For this review, take the finished solid that the model builds, in its own axes (mm). Face numbers are marked on the shaded views. A direction names the side the tool comes from. Coordinates: 2 decimals unless noted, no trailing zeros.
1. Machinability: for the marked faces 1 and 2, which of the approach directions +Z, -Z, +X, -X, +Y, -Y give a long, thin tool a straight path to every point of the face, cutting with its end or side? Answer none if there is none.
2. Clearance check with flat-ended pins moving along their axes: P1, Ø12, axis at y = -27, z = -39.5, coming from the +X side; P2, Ø1.5, axis at y = -68, z = 23, coming from the +X side; P3, Ø1.2, axis at y = 6.5, z = 12, coming from the +X side; P4, Ø12, axis at x = 10, z = -38.5, coming from the -Y side. State where each tip first meets the part, or that it passes through.
3. Mouldability with a two-part tool opening along Y and no side actions: class the marked faces 3 and 4 as pulls with the +Y half, pulls with the -Y half, needs draft (parallel to the pull), parting line crosses it, or undercut.
4. To check wall thickness, follow probe 1 along X at (y, z) = (51.5, -46.5); probe 2 along Y at (x, z) = (-2, -27); probe 3 along Z at (x, y) = (-1, 8.5). State the ranges of each line that lie inside material, in increasing order.
5. Take a section at A-A, the plane y = -26. Count the separate pieces of the cut face and the enclosed holes in it, then the cut area to 3 significant figures.
```python
from build123d import *

# Parameters (mm, degrees)
F0_R     = 85
F0_R_2   = 60.1341050947
F1_DEPTH = 10
F0_R_3   = 5
F0_R_4   = 18.4571799951
F2_DEPTH = 2.5
F3_DEPTH = 10
F4_R     = 5
F0_R_5   = 7.4694808043
F6_DEPTH = 20


# Not quite as in the source:
# - a fillet or chamfer that OpenCascade refuses, or shapes differently, is made with other operations: its cross-section is extruded or revolved along the edge and cut away or added


with BuildPart() as f1:
    # F0 (on Right) → F1 (new body, symmetric)
    with BuildSketch(Plane.YZ):
        Circle(F0_R)
        Circle(F0_R_2, mode=Mode.SUBTRACT)
    extrude(amount=F1_DEPTH, both=True)

    # F0 (on Right) → F2 (join, symmetric)
    with BuildSketch(Plane.YZ):
        Circle(F0_R_2)
        with Locations((-25.7258657366, -25.725863874)):
            Circle(F0_R_3, mode=Mode.SUBTRACT)
        with Locations((26.0370634496, -26.0024871677)):
            Circle(F0_R_3, mode=Mode.SUBTRACT)
        with Locations((-26, 26)):
            Circle(F0_R_3, mode=Mode.SUBTRACT)
        Circle(F0_R_4, mode=Mode.SUBTRACT)
        with Locations((26.2791067362, 26.2791085988)):
            Circle(F0_R_3, mode=Mode.SUBTRACT)
    extrude(amount=F2_DEPTH, both=True)

    # F0 (on Right) → F3 (join, symmetric)
    with BuildSketch(Plane.YZ):
        Circle(F0_R_4)
        Polygon((12.8988242803, 8.4499999602), (13.7673267676, -6.9457095256), (0.8685024874, -15.3957094858), (-12.8988242803, -8.4499999602), (-13.7673267676, 6.9457095256), (-0.8685024874, 15.3957094858), align=None, mode=Mode.SUBTRACT)
    extrude(amount=F3_DEPTH, both=True)

    # F4
    f4_edges = [f1.edges().sort_by_distance(p)[0] for p in [
        (-10, -85, 0),
        (10, -85, 0),
    ]]
    fillet(f4_edges, radius=F4_R)

    # F5: chamfer of 5 on 2 edges, made by hand

    # F5_s1 → F5_t2 (revolve, cut)
    with BuildSketch(Plane.XY):
        Polygon((5, 18.4571799951), (10, 13.4571799951), (10, 18.4571799951), align=None)
    revolve(axis=Axis((10, 0, 0), (1, 0, 0)), mode=Mode.SUBTRACT)

    # F5_s3 → F5_t4 (revolve, cut)
    with BuildSketch(Plane.XY):
        Polygon((-5, 18.4571799951), (-10, 13.4571799951), (-10, 18.4571799951), align=None)
    revolve(axis=Axis((-10, 0, 0), (1, 0, 0)), mode=Mode.SUBTRACT)

    # F0 (on Right) → F6 (join)
    with BuildSketch(Plane.YZ):
        Polygon((0.8685024874, -15.3957094858), (13.7673267676, -6.9457095256), (12.8988242803, 8.4499999602), (-0.8685024874, 15.3957094858), (-13.7673267676, 6.9457095256), (-12.8988242803, -8.4499999602), align=None)
        Circle(F0_R_5, mode=Mode.SUBTRACT)
    extrude(amount=F6_DEPTH)


solid = f1.part
```
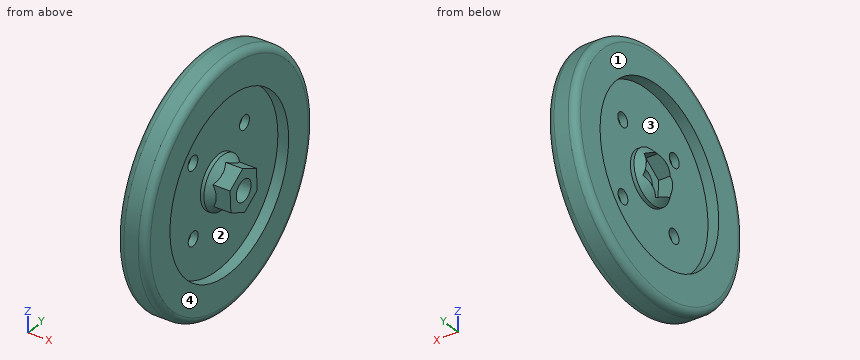
Results list:
1. face 1: +Z, -Z, -X, +Y, -Y
1. face 2: +X
2. P1: stops at x = 2.5
2. P2: stops at x = 10
2. P3: stops at x = 20
2. P4: stops at y = -77.82
3. face 3: undercut
3. face 4: needs draft
4. probe 1: x = -10 to 10
4. probe 2: y = -80.6 to -30.56, -20.89 to 21.14, 30.94 to 80.6
4. probe 3: z = -84.57 to -10.4, 10.67 to 84.57
5. separate pieces: 3
5. enclosed holes: 0
5. area: 1,490 mm2
